Verification items for the finished model (mm, model axes). Face numbers are marked on the shaded views. A direction names the side the tool comes from. Coordinates: 2 decimals unless noted, no trailing zeros. Order: outer loops, then holes, each group sorted by start corner. A loop starts at its lowest first (then second) coordinate and runs counter-clockwise, first axis right, second up. Notation, with made-up numbers: M 48.5,46 L 60.5,46 A18 cw 60.5,76 Z; hole C 27,62 d5. An arc over 180 degrees is marked long. Return JSON: item names as keys, results as strings. Group by question number.
Q1. Access from +Z, -Z, +X, -X, +Y, -Y to the whole of each face (thin tool, end or side, straight path). Record for the marked faces 4, 5 and 6.
Q2. Section check D-D, the plane z = 63. Enter the section's corners in (x, y), then the cut area to 3 significant figures.
Q3. Section check C-C, the plane x = -48. Enter the section's corners in (y, z).
Q4. Section check B-B, the plane y = 49.5. Enter the section's corners in (x, z).
Q5. Thickness scan on probe 1 along X at (y, z) = (136, 0); probe 2 along X at (y, z) = (87, 0); probe 3 along X at (y, z) = (120.5, -20). Record the ranges inside material, lowest first.
Q6. Mould release check, pull along X, two halves, no side actions. Record for the marked faces 1, 2 and 3: pulls with the +X half, pulls with the -X half, needs draft (parallel to the pull), parting line crosses it, or undercut.
Q7. Go/stop test with flat-tipped pins: pin 1 Ø6 at (x, y) = (-6.5, 17.5) entering from -Z; pin 2 Ø10 at (x, z) = (29, -66.5) entering from +Y; pin 3 Ø2.5 at (y, z) = (77, 16.5) entering from +X. Record where each tip stops, or that it passes through.
Q8. Section check A-A, the plane y = 94.5. Enter the section's corners in (x, z).
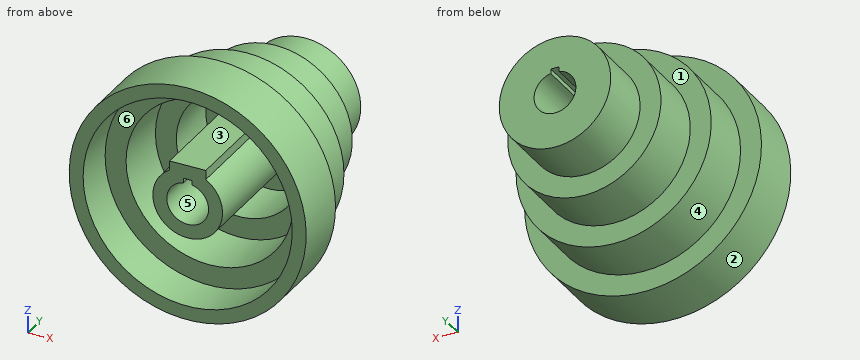
from build123d import *

# Parameters (mm, degrees)
SKETCH1_R            = 85
BOSS_EXTRUDE1_DEPTH  = 40
SKETCH2_R            = 70
BOSS_EXTRUDE2_DEPTH  = 40
SKETCH3_R            = 55
BOSS_EXTRUDE3_DEPTH  = 40
SKETCH4_R            = 40
BOSS_EXTRUDE4_DEPTH  = 40
SKETCH5_R            = 15
SKETCH5_W            = 6
SKETCH5_H            = 6
CUT_EXTRUDE1_DEPTH   = 201.124960962
SHELL1_OUTLINE_R     = 60
SHELL1_DEPTH         = 70
SHELL1_2_OUTLINE_R   = 75
SHELL1_2_OUTLINE_R_2 = 60
SHELL1_2_DEPTH       = 30
SHELL1_START         = 70
SHELL1_3_OUTLINE_R   = 45
SHELL1_3_DEPTH       = 40
SHELL1_START_2       = 110
SHELL1_4_DEPTH       = 40


# Read off the part's stored shape, not the designer's step: Shell1
with BuildPart() as part:
    # Sketch1 → Boss-Extrude1 (new body)
    with BuildSketch(Plane(origin=(0, 0, 0), x_dir=(1, 0, 0), z_dir=(0, 1, 0))):
        with Locations(Location((0, 0, 0), (0, 0, 270))):
            Circle(SKETCH1_R)
    extrude(amount=BOSS_EXTRUDE1_DEPTH)

    # Sketch2 → Boss-Extrude2 (add)
    with BuildSketch(Plane(origin=(0, 40, 0), x_dir=(1, 0, 0), z_dir=(0, 1, 0))):
        with Locations(Location((0, 0, 0), (0, 0, 270))):
            Circle(SKETCH2_R)
    extrude(amount=BOSS_EXTRUDE2_DEPTH)

    # Sketch3 → Boss-Extrude3 (add)
    with BuildSketch(Plane(origin=(0, 80, 0), x_dir=(1, 0, 0), z_dir=(0, 1, 0))):
        with Locations(Location((0, 0, 0), (0, 0, 270))):
            Circle(SKETCH3_R)
    extrude(amount=BOSS_EXTRUDE3_DEPTH)

    # Sketch4 → Boss-Extrude4 (add)
    with BuildSketch(Plane(origin=(0, 120, 0), x_dir=(1, 0, 0), z_dir=(0, 1, 0))):
        with Locations(Location((0, 0, 0), (0, 0, 270))):
            Circle(SKETCH4_R)
    extrude(amount=BOSS_EXTRUDE4_DEPTH)

    # Sketch5 → Cut-Extrude1 (cut, through all)
    with BuildSketch(Plane(origin=(0, 160, 0), x_dir=(1, 0, 0), z_dir=(0, 1, 0))):
        Circle(SKETCH5_R)
        with Locations((0, -15)):
            Rectangle(SKETCH5_W, SKETCH5_H)
    extrude(amount=-CUT_EXTRUDE1_DEPTH, mode=Mode.SUBTRACT)

    # Shell1 outline → Shell1 (cut)
    with BuildSketch(Plane(origin=(0, 0, 0), x_dir=(1, 0, 0), z_dir=(0, 1, 0))):
        Circle(SHELL1_OUTLINE_R)
        with BuildLine():
            Line((13, -21.354156504), (13, -28))
            Line((13, -28), (-13, -28))
            Line((-13, -28), (-13, -21.354156504))
            ThreePointArc((-13, -21.354156504), (0, 25), (13, -21.354156504))
        make_face(mode=Mode.SUBTRACT)
    extrude(amount=SHELL1_DEPTH, mode=Mode.SUBTRACT)

    # Shell1 2 outline → Shell1 2 (cut)
    with BuildSketch(Plane(origin=(0, 0, 0), x_dir=(1, 0, 0), z_dir=(0, 1, 0))):
        Circle(SHELL1_2_OUTLINE_R)
        Circle(SHELL1_2_OUTLINE_R_2, mode=Mode.SUBTRACT)
    extrude(amount=SHELL1_2_DEPTH, mode=Mode.SUBTRACT)

    # Shell1 3 outline → Shell1 3 (cut)
    with BuildSketch(Plane(origin=(0, 0, 0), x_dir=(1, 0, 0), z_dir=(0, 1, 0)).offset(SHELL1_START)):
        Circle(SHELL1_3_OUTLINE_R)
        with BuildLine():
            Line((13, -21.354156504), (13, -28))
            Line((13, -28), (-13, -28))
            Line((-13, -28), (-13, -21.354156504))
            ThreePointArc((-13, -21.354156504), (0, 25), (13, -21.354156504))
        make_face(mode=Mode.SUBTRACT)
    extrude(amount=SHELL1_3_DEPTH, mode=Mode.SUBTRACT)

    # Shell1 4 outline → Shell1 4 (cut)
    with BuildSketch(Plane(origin=(0, 0, 0), x_dir=(1, 0, 0), z_dir=(0, 1, 0)).offset(SHELL1_START_2)):
        with BuildLine():
            Line((13, -21.354156504), (13, -27.037011669))
            ThreePointArc((13, -27.037011669), (0, 30), (-13, -27.037011669))
            Line((-13, -27.037011669), (-13, -21.354156504))
            ThreePointArc((-13, -21.354156504), (0, 25), (13, -21.354156504))
        make_face()
        with BuildLine():
            ThreePointArc((-10.770329614, -28), (0, -30), (10.770329614, -28))
            Line((10.770329614, -28), (-10.770329614, -28))
        make_face()
    extrude(amount=SHELL1_4_DEPTH, mode=Mode.SUBTRACT)


solid = part.part
Numbers:
{
 "1": {"face 4": "+Y", "face 5": "+Y, -Y", "face 6": "-Y"},
 "2": {"outline": "M -57.06,0 L -40.69,0 L -40.69,30 L 40.69,30 L 40.69,0 L 57.06,0 L 57.06,40 L 30.51,40 L 30.51,80 L -30.51,80 L -30.51,40 L -57.06,40 Z", "area": "4,560 mm2"},
 "3": {"outline": "M 0,-70.15 L 40,-70.15 L 40,-50.95 L 80,-50.95 L 80,-26.85 L 120,-26.85 L 120,26.85 L 80,26.85 L 80,50.95 L 40,50.95 L 40,70.15 L 0,70.15 L 0,57.63 L 30,57.63 L 30,36 L 70,36 L 70,-36 L 30,-36 L 30,-57.63 L 0,-57.63 Z"},
 "4": {"outline": "C 0,0 d140; M -13,21.35 A25 ccw long 13,21.35 L 13,28 L -13,28 Z; hole C 0,0 d120; hole M -3,14.7 A15 ccw long 3,14.7 L 3,18 L -3,18 Z"},
 "5": {"probe 1": "x = -40 to -30, -25 to -15, 15 to 25, 30 to 40", "probe 2": "x = -55 to -45, -25 to -15, 15 to 25, 45 to 55", "probe 3": "x = -34.64 to -22.36, -15 to 15, 22.36 to 34.64"},
 "6": {"face 1": "needs draft", "face 2": "parting line crosses it", "face 3": "undercut"},
 "7": {"pin 1": "stops at z = -84.93", "pin 2": "stops at y = 80", "pin 3": "stops at x = 68.32"},
 "8": {"outline": "C 0,0 d110; M -13,21.35 A25 ccw long 13,21.35 L 13,28 L -13,28 Z; hole C 0,0 d90; hole M -3,14.7 A15 ccw long 3,14.7 L 3,18 L -3,18 Z"}
}
